from build123d import *

# Parameters (mm, degrees)
F1_DEPTH   = 504
F2_C1_SIZE = 9.9999
F2_C2_SIZE = 9.9999


# Not quite as in the source:
# - a fillet or chamfer is up to 0.001 mm smaller than in the source, because OpenCascade refuses the exact size


with BuildPart() as f1:
    # F0 (on Top) → F1 (new body)
    with BuildSketch(Plane.XY):
        Polygon((-3, 5), (-5, 5), (-5, -5), (5, -5), (5, 5), (3, 5), (3, -3), (-3, -3), align=None)
    extrude(amount=F1_DEPTH)

    # F2: chamfer of 10 on 4 edges, made by hand

    # F2_c1 (size 10 in the source; OpenCascade refuses exactly that, so slightly less here)
    f2_c1_edges = [f1.edges().sort_by_distance(p)[0] for p in [
        (-4, 5, 0),
    ]]
    chamfer(f2_c1_edges, length=F2_C1_SIZE)

    # F2_c2 (size 10 in the source; OpenCascade refuses exactly that, so slightly less here)
    f2_c2_edges = [f1.edges().sort_by_distance(p)[0] for p in [
        (-4, 5, 504),
    ]]
    chamfer(f2_c2_edges, length=F2_C2_SIZE)


solid = f1.part
Part model, mm, in its own coordinate system. A direction names the side the tool comes from. Round coordinates to 2 decimals unless told otherwise and drop trailing zeros. Write each loop counter-clockwise with the first axis right and the second up, starting at its lowest first coordinate (ties: lowest second). Pieces come first, ordered by that corner, then holes. Notation, with made-up numbers: (50.25, 87.5) - (72.25, 87.5) arc R12 ccw to (72.25, 104.5) - close; hole circle Ø2 at (29, 65.5). An arc over 180 degrees is marked (long way). Use CSV: the item, a comma, the result in double quotes.
Item 1: Slice it at A-A, the plane y = -1. Write the cut outline in (x, z), then the cut area to 3 significant figures.
Results list:
outline,"(-5, 4) - (-3, 4) - (-3, 500) - (-5, 500) - close; (3, 4) - (5, 4) - (5, 500) - (3, 500) - close"
area,"1,980 mm²"
Item 2: Flat gauge pins, fed straight in: P1, Ø3, axis at x = 0, z = 192.5, coming from the +Y side; P2, Ø4, axis at x = -4, y = -1.5, coming from the -Z side; P3, Ø5, axis at x = 2, y = 3, coming from the +Z side. Where does each tip first touch, or does it go through?
Results list:
P1,"stops at y = -3"
P2,"stops at z = 1.5"
P3,"stops at z = 498.29"
Item 3: Tool access for faces 1 (the flat face through (3.4, -1.2, 500.2)), 2 (the flat face through (3, 1, 248)): list every direction of +Z, -Z, +X, -X, +Y, -Y with a clear straight run to the whole face (end or side of a thin tool).
Results list:
face 1,"+Z, +X, -X, +Y"
face 2,"+Z, -Z, +Y"
Item 4: Pull direction X, two halves, no side cores. Call faces 3 (the flat face through (-3, 1, 248)), 4 (the flat face through (5, 0, 248)), 5 (the flat face through (3.4, -1.2, 3.8)), 6 (the flat face through (-5, 0, 248)): pulls with the +X half, pulls with the -X half, needs draft (parallel to the pull), parting line crosses it, or undercut.
Results list:
face 3,"undercut"
face 4,"pulls with the +X half"
face 5,"needs draft"
face 6,"pulls with the -X half"
Item 5: Slice it at B-B, the plane z = 431.5. Write the cut outline in (x, y).
Results list:
outline,"(-5, -5) - (5, -5) - (5, 5) - (3, 5) - (3, -3) - (-3, -3) - (-3, 5) - (-5, 5) - close"
Item 6: Wall check: L1, parallel to X at y = 2.5, z = 177.5; L2, parallel to Y at x = -0.5, z = 429.5; L3, parallel to Z at x = -3.5, y = -1.5. Give the ranges that are in metal, low to high.
Results list:
L1,"x = -5 to -3, 3 to 5"
L2,"y = -5 to -3"
L3,"z = 3.5 to 500.5"
